Part print with two shaded views. Sizes in mm from the minimum x, y, z corner. A direction names the side the tool comes from. Round coordinates to 2 decimals unless told otherwise and drop trailing zeros. Order: outer loops, then holes, each group sorted by start corner. A loop starts at its lowest first (then second) coordinate and runs counter-clockwise, first axis right, second up. Notation, with made-up numbers: (23.5, -1.75) - (45.5, -1.75) arc R27 cw to (45.5, 21.25) - close; hole circle Ø3 at (88, 89.25). An arc over 180 degrees is marked (long way). Write item = value, one per line.
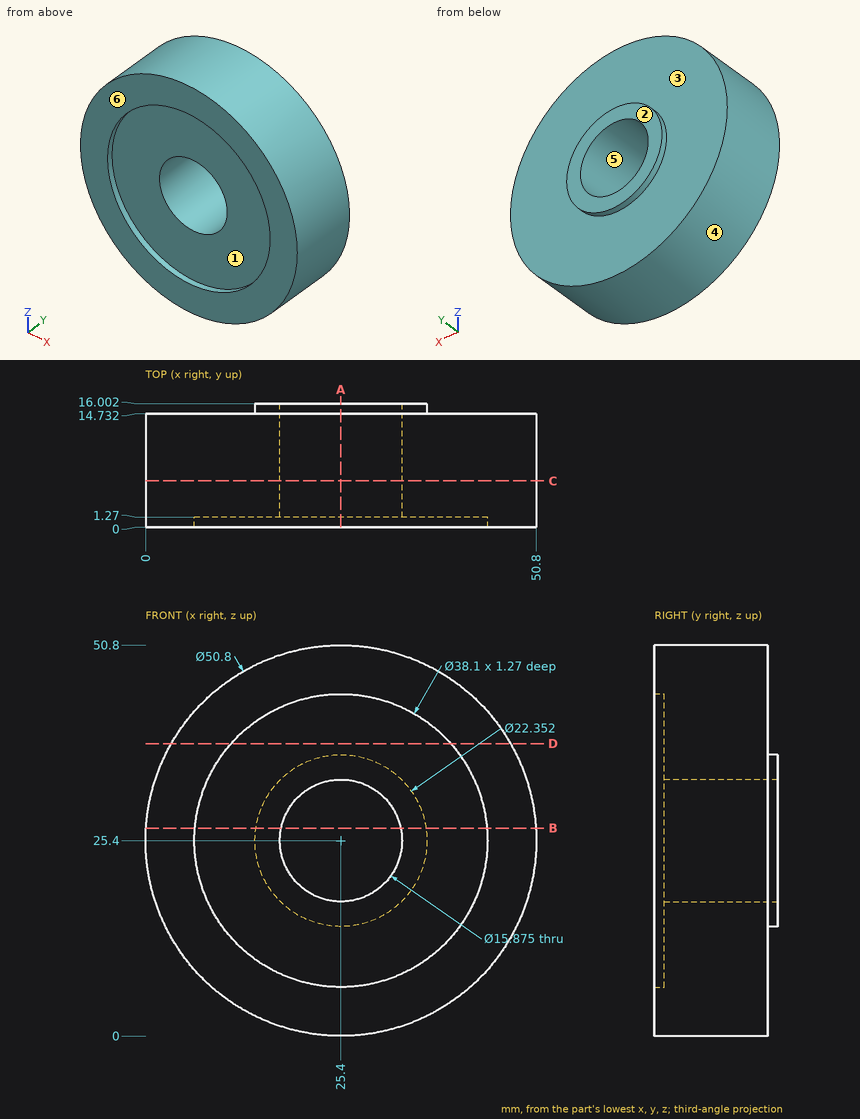
1) Flat gauge pins, fed straight in: pin 1 Ø8 at (x, y) = (27, 7.5) entering from -Z; pin 2 Ø6 at (x, y) = (7, 8.5) entering from +Z; pin 3 Ø2 at (y, z) = (4, 29.5) entering from +X. Where does each tip first touch, or does it go through?
Conclusion:
pin_1 = 0
pin_2 = 45.6
pin_3 = 50.61
2) Mould opens along Z. For the marked faces 4, 5 and 6 say: +Z half, -Z half, draft (parallel to the pull), parting line (faces both ways), or undercut.
Conclusion:
face_4 = parting line
face_5 = undercut
face_6 = draft
3) 3-axis set-ups, long thin cutter, end or side, ignore diameter. For the marked faces 1, 2 and 3: which of +Z, -Z, +X, -X, +Y, -Y reach the whole face in a straight line?
Conclusion:
face_1 = -Y
face_2 = +Z, -Z, +X, -X, +Y
face_3 = +Y
4) Cut at C-C (y = 6). Write the cut outline in (x, z) (1 decimal).
Conclusion:
outline = circle Ø50.8 at (25.4, 25.4); hole circle Ø15.9 at (25.4, 25.4)
5) Cut at A-A (x = 25.4). Write the cut outline in (y, z), and give its area (3 significant figures).
Conclusion:
outline = (0, 0) - (14.73, 0) - (14.73, 14.22) - (16, 14.22) - (16, 17.46) - (1.27, 17.46) - (1.27, 6.35) - (0, 6.35) - close; (0, 44.45) - (1.27, 44.45) - (1.27, 33.34) - (16, 33.34) - (16, 36.58) - (14.73, 36.58) - (14.73, 50.8) - (0, 50.8) - close
area = 495 mm^2
6) Cut at D-D (z = 38). Write the cut outline in (x, y), and give its area (3 significant figures).
Conclusion:
outline = (3.35, 0) - (11.11, 0) - (11.11, 1.27) - (39.69, 1.27) - (39.69, 0) - (47.45, 0) - (47.45, 14.73) - (3.35, 14.73) - close
area = 614 mm^2
7) Wall check: line 1 along Z through (x, y) = (25.4, 0.9); line 2 along X through (y, z) = (12.5, 25.4). Give the ranges that are in metal, low to high.
Conclusion:
line_1 = 0 to 6.35, 44.45 to 50.8
line_2 = 0 to 17.46, 33.34 to 50.8
8) Cut at B-B (z = 27). Write the cut outline in (x, y).
Conclusion:
outline = (0.05, 0) - (6.42, 0) - (6.42, 1.27) - (17.63, 1.27) - (17.63, 16) - (14.34, 16) - (14.34, 14.73) - (0.05, 14.73) - close; (33.17, 1.27) - (44.38, 1.27) - (44.38, 0) - (50.75, 0) - (50.75, 14.73) - (36.46, 14.73) - (36.46, 16) - (33.17, 16) - close
